For this review, take the finished solid that the model builds, in its own axes (mm). A direction names the side the tool comes from. Coordinates: 2 decimals unless noted, no trailing zeros. Loops run counter-clockwise (first coordinate to the right, second up) from the corner with the lowest first, then second, coordinate; pieces in that order, holes last. Notation, with made-up numbers: M 80.25,41 L 120.25,41 A18 ccw 120.25,52 Z; hole C 7,38.25 d8. An arc over 180 degrees is marked long. Write item = value, one per line.
from build123d import *

# Parameters (mm, degrees)
SKETCH_1_W          = 20
SKETCH_1_H          = 20
EXTRUDE_1_DEPTH     = 100
SKETCH_2_R          = 2.15
SKETCH_2_R_2        = 2
CUT_EXTRUDE_1_DEPTH = 101.995049384


with BuildPart() as part:
    # 스케치1 → 보스-돌출1 (new body)
    with BuildSketch(Plane.XY):
        Rectangle(SKETCH_1_W, SKETCH_1_H)
    extrude(amount=EXTRUDE_1_DEPTH)

    # 스케치2 → 컷-돌출1 (cut, through all)
    with BuildSketch(Plane.XY.offset(100)):
        Circle(SKETCH_2_R)
        with Locations((-7, 7)):
            Circle(SKETCH_2_R_2)
        with Locations((7, 7)):
            Circle(SKETCH_2_R_2)
        with Locations((7, -7)):
            Circle(SKETCH_2_R_2)
        with Locations((-7, -7)):
            Circle(SKETCH_2_R_2)
        with BuildLine():
            Line((-2.65, 10), (-2.65, 8.5))
            Line((-2.65, 8.5), (-4.15, 8.5))
            Line((-4.15, 8.5), (-4.15, 5.5))
            ThreePointArc((-4.15, 5.5), (0, 4), (4.15, 5.5))
            Line((4.15, 5.5), (4.15, 8.5))
            Line((4.15, 8.5), (2.65, 8.5))
            Line((2.65, 8.5), (2.65, 10))
            Line((2.65, 10), (-2.65, 10))
        make_face()
        with BuildLine():
            Line((10, 2.65), (8.5, 2.65))
            Line((8.5, 2.65), (8.5, 4.15))
            Line((8.5, 4.15), (5.5, 4.15))
            ThreePointArc((5.5, 4.15), (4, 0), (5.5, -4.15))
            Line((5.5, -4.15), (8.5, -4.15))
            Line((8.5, -4.15), (8.5, -2.65))
            Line((8.5, -2.65), (10, -2.65))
            Line((10, -2.65), (10, 2.65))
        make_face()
        with BuildLine():
            Line((2.65, -10), (2.65, -8.5))
            Line((2.65, -8.5), (4.15, -8.5))
            Line((4.15, -8.5), (4.15, -5.5))
            ThreePointArc((4.15, -5.5), (0, -4), (-4.15, -5.5))
            Line((-4.15, -5.5), (-4.15, -8.5))
            Line((-4.15, -8.5), (-2.65, -8.5))
            Line((-2.65, -8.5), (-2.65, -10))
            Line((-2.65, -10), (2.65, -10))
        make_face()
        with BuildLine():
            Line((-10, -2.65), (-8.5, -2.65))
            Line((-8.5, -2.65), (-8.5, -4.15))
            Line((-8.5, -4.15), (-5.5, -4.15))
            ThreePointArc((-5.5, -4.15), (-4, 0), (-5.5, 4.15))
            Line((-5.5, 4.15), (-8.5, 4.15))
            Line((-8.5, 4.15), (-8.5, 2.65))
            Line((-8.5, 2.65), (-10, 2.65))
            Line((-10, 2.65), (-10, -2.65))
        make_face()
    extrude(amount=-CUT_EXTRUDE_1_DEPTH, mode=Mode.SUBTRACT)


solid = part.part
Q1. Add section A-A (y = -7). Write out the cut boundary in (x, z), and give its area (3 significant figures).
Solved:
outline = M -10,0 L -9,0 L -9,100 L -10,100 Z; M -5,0 L -4.15,0 L -4.15,100 L -5,100 Z; M 4.15,0 L 5,0 L 5,100 L 4.15,100 Z; M 9,0 L 10,0 L 10,100 L 9,100 Z
area = 370 mm²
Q2. Add section C-C (y = 0). Write out the cut boundary in (x, z).
Solved:
outline = M -4,0 L -2.15,0 L -2.15,100 L -4,100 Z; M 2.15,0 L 4,0 L 4,100 L 2.15,100 Z
Q3. Machinability: for faces 1 (the face through (6, 10, 49)), 2 (the face through (-4.15, 7, 51)), which of the approach directions +Z, -Z, +X, -X, +Y, -Y give a long, thin tool a straight path to every point of the face, cutting with its end or side? Answer none if there is none.
Solved:
face_1 = +Z, -Z, +X, -X, +Y
face_2 = +Z, -Z
Q4. Draft analysis for pull direction X (two halves, no side actions). For faces 3 (the face through (10, -6, 49)), 4 (the face through (-0.1, 2.4, 100)), 5 (the face through (4, 0, 51)), state which applies: +X half, -X half, draft (parallel to the pull), parting line (faces both ways), or undercut.
Solved:
face_3 = +X half
face_4 = draft
face_5 = undercut
Q5. For pin 1 Ø1.5 at (x, y) = (-2.5, 7.5) entering from -Z, flat-tipped, find the tip position at first contact; note if it passes through.
Solved:
pin_1 = through
Q6. For line 1 along Y through (x, z) = (7, 79.5); line 2 along X through (y, z) = (6, 21); line 3 along Y through (x, z) = (-3.5, 86), list the stretches that pass through material, from the lowest coordinate up.
Solved:
line_1 = -10 to -9, -5 to -4.15, 4.15 to 5, 9 to 10
line_2 = -10 to -8.73, -5.27 to -4.15, 4.15 to 5.27, 8.73 to 10
line_3 = -10 to -8.5, -5.02 to 5.02, 8.5 to 10
